from build123d import *

# Parameters (mm, degrees)
SKETCH1_W                = 140.9
SKETCH1_H                = 80
PCB_DEPTH                = 1.55
BODYC_DEPTH              = 0.4
BODYC_DEPTH_BACK         = 6.45
BOSS_EXTRUDE4_DEPTH      = 7.1
BOSS_EXTRUDE4_DEPTH_BACK = 1.55
SKETCH4_W                = 13.65
SKETCH4_H                = 13.15
SKETCH5_W                = 4.65
SKETCH5_H                = 3.1
CUT_EXTRUDE3_DEPTH       = 14.1
SKETCH11_W               = 24.15
SKETCH11_H               = 1.55
BOSS_EXTRUDE8_DEPTH      = 29
SKETCH7_W                = 24.15
SKETCH7_H                = 1.55
BOSS_EXTRUDE5_DEPTH      = 29
CUT_EXTRUDE4_DEPTH       = 89
SKETCH12_R               = 9.15
BATTERY_DEPTH            = 54
SKETCH13_R               = 1
BUTTON_DEPTH             = 1.3
SKETCH14_R               = 1
RESET_DEPTH              = 1.3


with BuildPart() as part:
    # Sketch1 → PCB (new body)
    with BuildSketch(Plane(origin=(0, 0, 0), x_dir=(1, 0, 0), z_dir=(0, 1, 0))):
        Rectangle(SKETCH1_W, SKETCH1_H)
    extrude(amount=PCB_DEPTH)

    # Sketch3 → bodyC (add, two sides: drawn at the far end of the back side and taken through both)
    with BuildSketch(Plane.ZY.offset(70.45).offset(-BODYC_DEPTH_BACK)):
        with BuildLine():
            Line((-34.3, 4.75), (-28.56, 4.75))
            ThreePointArc((-28.56, 4.75), (-26.96, 3.15), (-28.56, 1.55))
            Line((-28.56, 1.55), (-34.3, 1.55))
            ThreePointArc((-34.3, 1.55), (-35.9, 3.15), (-34.3, 4.75))
        make_face()
    extrude(amount=BODYC_DEPTH + BODYC_DEPTH_BACK)

    # Sketch4 → Boss-Extrude4 (add, two sides: drawn at the far end of the back side and taken through both)
    with BuildSketch(Plane(origin=(0, 1.55, 0), x_dir=(1, 0, 0), z_dir=(0, 1, 0)).offset(-BOSS_EXTRUDE4_DEPTH_BACK)):
        with Locations((-68.275, 17.575)):
            Rectangle(SKETCH4_W, SKETCH4_H)
    extrude(amount=BOSS_EXTRUDE4_DEPTH + BOSS_EXTRUDE4_DEPTH_BACK)

    # Sketch5 → Cut-Extrude3 (cut)
    with BuildSketch(Plane.XY.offset(-11)):
        with Locations((-72.775, 1.55)):
            Rectangle(SKETCH5_W, SKETCH5_H)
    extrude(amount=-CUT_EXTRUDE3_DEPTH, mode=Mode.SUBTRACT)

    # Sketch11 → Boss-Extrude8 (add)
    with BuildSketch(Plane(origin=(0, 1.55, 0), x_dir=(1, 0, 0), z_dir=(0, 1, 0))):
        with Locations((-32.275, 27.625)):
            Rectangle(SKETCH11_W, SKETCH11_H)
    extrude(amount=BOSS_EXTRUDE8_DEPTH)

    # Sketch7 → Boss-Extrude5 (add)
    with BuildSketch(Plane(origin=(0, 1.55, 0), x_dir=(1, 0, 0), z_dir=(0, 1, 0))):
        with Locations((-32.275, -27.325)):
            Rectangle(SKETCH7_W, SKETCH7_H)
    extrude(amount=BOSS_EXTRUDE5_DEPTH)

    # Sketch8 → Cut-Extrude4 (cut)
    with BuildSketch(Plane.XY.offset(28.1)):
        Polygon((-44.35, 30.55), (-20.2, 22.85), (-20.2, 30.55), align=None)
    extrude(amount=-CUT_EXTRUDE4_DEPTH, mode=Mode.SUBTRACT)

    # Sketch12 → Battery (add)
    with BuildSketch(Plane.XY.offset(-26.85)):
        with Locations(Location((-32.275, 12.25, 0), (0, 0, 180))):
            Circle(SKETCH12_R)
    extrude(amount=BATTERY_DEPTH)

    # Sketch13 → Button (add)
    with BuildSketch(Plane(origin=(0, 1.55, 0), x_dir=(1, 0, 0), z_dir=(0, 1, 0))):
        with Locations(Location((-62.75, -28.6, 0), (0, 0, 90))):
            Circle(SKETCH13_R)
    extrude(amount=BUTTON_DEPTH)

    # Sketch14 → Reset (add)
    with BuildSketch(Plane(origin=(0, 1.55, 0), x_dir=(1, 0, 0), z_dir=(0, 1, 0))):
        with Locations(Location((-25.75, 9.9, 0), (0, 0, 90))):
            Circle(SKETCH14_R)
    extrude(amount=RESET_DEPTH)


solid = part.part
For this review, take the finished solid that the model builds, in its own axes (mm). A direction names the side the tool comes from. Round coordinates to 2 decimals unless told otherwise and drop trailing zeros. Write each loop counter-clockwise with the first axis right and the second up, starting at its lowest first coordinate (ties: lowest second). Pieces come first, ordered by that corner, then holes. Notation, with made-up numbers: M -7,-14.75 L 11,-14.75 A20 ccw 11,-3.75 Z; hole C -34,-33.5 d3. An arc over 180 degrees is marked long. Write item = value, one per line. Start each with the question number.
(1) Clearance check with flat-ended pins moving along their axes: pin 1 Ø2 at (x, z) = (-62.5, 28.5) entering from +Y; pin 2 Ø10 at (y, z) = (4.5, 1.5) entering from +X; pin 3 Ø1 at (y, z) = (7.5, 8) entering from -X; pin 4 Ø5 at (y, z) = (7, 10) entering from -X. State where each tip first meets the part, or that it passes through.
(2) We need section C-C (y = 25). Give the boundary of the cut face in (x, z), then the cut area to 3 significant figures.
(3) For line 1 along Y through (x, z) = (55.5, -26.5); line 2 along X through (y, z) = (4.5, -12.5); line 3 along Z through (x, y) = (-36.5, 14), list the stretches that pass through material, from the lowest coordinate up.
(4) We need section A-A (z = 25). Give the boundary of the cut face in (x, y) (3 decimals).
(5) The part is to be moulded in two halves that separate along Z. For faces 1 (the face through (-75.1, 6, -17)), 2 (the face through (-32, 22, 26.55)), 3 (the face through (-32, 13, 28.1)), say which applies: +Z half, -Z half, draft (parallel to the pull), parting line (faces both ways), or undercut.
(6) We need section B-B (y = 12.25). Give the boundary of the cut face in (x, z) (3 decimals).
(7) For faces 4 (the face through (-64, 3, -31)), 5 (the face through (-68, 5, -24.15)), 6 (the face through (-23.134, 11.848, -0.524)), list the 3-axis set-ups (+Z, -Z, +X, -X, +Y, -Y) from which the entire face can be reached by the end or side of a thin tool; tool diameter is ignored.
(8) We need section D-D (x = 22). Give the boundary of the cut face in (y, z), then the cut area to 3 significant figures.
Results found:
q1.pin_1 = 2.85
q1.pin_2 = 70.45
q1.pin_3 = -40.38
q1.pin_4 = -41
q2.outline = M -44.35,-28.4 L -26.94,-28.4 L -26.94,-26.85 L -44.35,-26.85 Z; M -44.35,26.55 L -26.94,26.55 L -26.94,28.1 L -44.35,28.1 Z
q2.area = 54.0 mm²
q3.line_1 = 0 to 1.55
q3.line_2 = -75.1 to -61.45, -37.14 to -27.41
q3.line_3 = -28.4 to 28.1
q4.outline = M -70.45,0 L 70.45,0 L 70.45,1.55 L -70.45,1.55 Z; C -32.275,12.25 d18.3
q5.face_1 = draft
q5.face_2 = undercut
q5.face_3 = +Z half
q6.outline = M -44.35,-28.4 L -20.2,-28.4 L -20.2,-26.85 L -23.125,-26.85 L -23.125,26.55 L -20.2,26.55 L -20.2,28.1 L -44.35,28.1 L -44.35,26.55 L -41.425,26.55 L -41.425,-26.85 L -44.35,-26.85 Z
q7.face_4 = -Z, +Y
q7.face_5 = -X, +Y
q7.face_6 = none
q8.outline = M 0,-40 L 1.55,-40 L 1.55,40 L 0,40 Z
q8.area = 124 mm²
